Source: CAD feature listing. Evaluate the final solid. Frame: model axes, mm. Face numbers are marked on the shaded views. Round coordinates to 2 decimals unless told otherwise and drop trailing zeros. Loops run counter-clockwise (first coordinate to the right, second up) from the corner with the lowest first, then second, coordinate; pieces in that order, holes last.
Item 1: Section query B-B on y = 2.75. Return loops of the section in (x, z), then the cut area to 3 significant figures.
Item 2: Section query D-D on z = 7.25. Return loops of the section in (x, y).
Item 3: Section query C-C on x = 2.8. Return loops of the section in (y, z).
Item 4: Section query A-A on z = 3.5. Return loops of the section in (x, y).
Item 5: Pull-direction query (Y, two-part tool) for the marked faces 1, 2, 3 and 4; classes: released by +Y, released by -Y, zero draft, split by the parting line, or undercut.
Item 6: Ray query, L1, parallel to X at y = 2.75, z = 6.25; L2, parallel to Y at x = 22.7, z = 2; L3, parallel to X at y = 2.75, z = 2.75. Return the intervals inside material, ascending.
Autodesk Inventor part; units mm, degrees
ref_plane "YZ Plane" through (0, 0, 0) normal (1, 0, 0) x (0, 1, 0)
ref_plane "XZ Plane" through (0, 0, 0) normal (0, 1, 0) x (-1, 0, 0)
ref_plane "XY Plane" through (0, 0, 0) normal (0, 0, 1) x (1, 0, 0)
sketch "Skizze1" plane through (0, 0, 0) normal (0, 1, 0) x (-1, 0, 0)
  line L0 (0, 0) -> (-25.5, 0)
  line L1 (-25.5, 0) -> (-25.5, 9)
  line L2 (-25.5, 9) -> (0, 9)
  line L3 (0, 9) -> (0, 0)
  dimension "d0" = 25.5
  dimension "d1" = 9
extrude "Extrusion1" add sketch "Skizze1" along normal blind 5.5
sketch "Skizze2" plane through (0, 0, 0) normal (0, -1, 0) x (1, 0, 0)
  line L0 (25.5, 0) -> (0, 0)
  arc A0 (18.75, 0) -> (6.75, 0) centre (12.75, 0) ccw
  dimension "d4" = 12
extrude "Extrusion2" cut sketch "Skizze2" against normal through all
sketch "Skizze5" plane through (0, 0, 9) normal (0, 0, 1) x (1, 0, 0)
  line L0 (0, 0) -> (0, 5.5) construction
  line L1 (0, 2.75) -> (25.5934, 2.75) construction
  line L2 (25.5, 0) -> (0, 0) construction
  line L3 (12.75, 0) -> (12.75, 5.5) construction
  line L4 (0, 5.5) -> (25.5, 5.5) construction
  point P0 (2.8, 2.75)
  point P1 (22.7, 2.75)
  dimension "d33" = 2.8
hole "Bohrung4" at (2.8, 2.75, 9) at (22.7, 2.75, 9) direction (0, 0, -1) diameter 3.3 end through all
fillet "Rundung1" radius 2 4 edges at (25.5, 0, 4.5) (25.5, 5.5, 4.5) (0, 0, 4.5) (0, 5.5, 4.5)
properties part number "Motorhalterung_oben" material "ABS-Kunststoff"
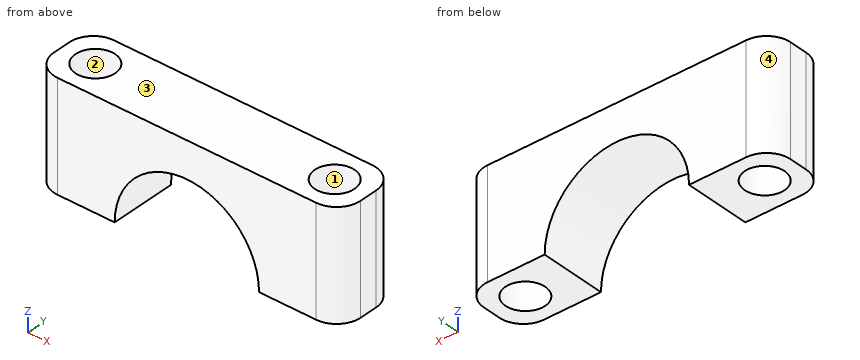
Data:
1. outline: (0, 0) - (1.15, 0) - (1.15, 9) - (0, 9) - close; (4.45, 0) - (6.75, 0) arc R6 cw to (18.75, 0) - (21.05, 0) - (21.05, 9) - (4.45, 9) - close; (24.35, 0) - (25.5, 0) - (25.5, 9) - (24.35, 9) - close
1. area: 114 mm2
2. outline: (0, 2) arc R2 ccw to (2, 0) - (23.5, 0) arc R2 ccw to (25.5, 2) - (25.5, 3.5) arc R2 ccw to (23.5, 5.5) - (2, 5.5) arc R2 ccw to (0, 3.5) - close; hole circle Ø3.3 at (2.8, 2.75); hole circle Ø3.3 at (22.7, 2.75)
3. outline: (0, 0) - (1.1, 0) - (1.1, 9) - (0, 9) - close; (4.4, 0) - (5.5, 0) - (5.5, 9) - (4.4, 9) - close
4. outline: (0, 2) arc R2 ccw to (2, 0) - (7.88, 0) - (7.88, 5.5) - (2, 5.5) arc R2 ccw to (0, 3.5) - close; (17.62, 0) - (23.5, 0) arc R2 ccw to (25.5, 2) - (25.5, 3.5) arc R2 ccw to (23.5, 5.5) - (17.62, 5.5) - close; hole circle Ø3.3 at (2.8, 2.75); hole circle Ø3.3 at (22.7, 2.75)
5. face 1: undercut
5. face 2: undercut
5. face 3: zero draft
5. face 4: released by +Y
6. L1: x = 0 to 1.15, 4.45 to 21.05, 24.35 to 25.5
6. L2: y = 0 to 1.1, 4.4 to 5.5
6. L3: x = 0 to 1.15, 4.45 to 7.42, 18.08 to 21.05, 24.35 to 25.5
